```python
from build123d import *

# Parameters (mm, degrees)
SKETCH2_W           = 109
SKETCH2_H           = 114
BOSS_EXTRUDE1_DEPTH = 1.5
SKETCH3_W           = 104
SKETCH3_H           = 109
BOSS_EXTRUDE2_DEPTH = 1
SKETCH4_W           = 25
SKETCH4_H           = 18
CUT_EXTRUDE1_DEPTH  = 2.5


with BuildPart() as part:
    # Sketch2 → Boss-Extrude1 (new body)
    with BuildSketch(Plane(origin=(0, 0, 0), x_dir=(1, 0, 0), z_dir=(0, 1, 0))):
        Rectangle(SKETCH2_W, SKETCH2_H)
    extrude(amount=BOSS_EXTRUDE1_DEPTH)

    # Sketch3 → Boss-Extrude2 (add)
    with BuildSketch(Plane(origin=(0, 1.5, 0), x_dir=(1, 0, 0), z_dir=(0, 1, 0))):
        Rectangle(SKETCH3_W, SKETCH3_H)
    extrude(amount=BOSS_EXTRUDE2_DEPTH)

    # Sketch4 → Cut-Extrude1 (cut)
    with BuildSketch(Plane(origin=(0, 2.5, 0), x_dir=(1, 0, 0), z_dir=(0, 1, 0))):
        with Locations((42, -40.5)):
            Rectangle(SKETCH4_W, SKETCH4_H)
    extrude(amount=-CUT_EXTRUDE1_DEPTH, mode=Mode.SUBTRACT)


solid = part.part
```
Geometry: final body of the model. Coordinates: model frame, mm. A direction names the side the tool comes from. Coordinates: 2 decimals unless noted, no trailing zeros. Loops run counter-clockwise (first coordinate to the right, second up) from the corner with the lowest first, then second, coordinate; pieces in that order, holes last. Notation, with made-up numbers: (53, 34) -> (107, 34) arc R18 ccw to (107, 64) -> close; hole circle Ø11 at (4.25, 9). An arc over 180 degrees is marked (long way). Use a Markdown table: item, result. Add a question column.
(1) Section query A-A, the plane x = 43.5. Return loops of the section in (y, z), plus the area to 3 significant figures.
(2) Section query D-D, the plane x = -2.5. Return loops of the section in (y, z).
(3) Section query B-B, the plane y = 0.7. Return loops of the section in (x, z).
(4) Mould query, pull axis Z, two halves, no side actions, for faces 1 (the flat face through (-53, 1.5, -4)), 2 (the flat face through (42, 1, 49.5)). Classes: pulls with the +Z half, pulls with the -Z half, needs draft (parallel to the pull), parting line crosses it, or undercut.
(5) Pin query (flat end, axial travel): pin 1 Ø0.8 at (x, y) = (37, 2) entering from +Z; pin 2 Ø0.5 at (y, z) = (2, 52.5) entering from +X; pin 3 Ø0.8 at (y, z) = (2, 4) entering from -X. Return the tip coordinate at first contact, or that it passes through.
(6) Section query C-C, the plane z = 37. Return loops of the section in (x, y).
(7) Line query: line 1 along Z through (x, y) = (43.5, 1.7); line 2 along Z through (x, y) = (34, 1.3); line 3 along X through (y, z) = (2.25, 26). Output: solid intervals per line, ascending.
(8) Access query for faces 3 (the flat face through (29.5, 1, 41)), 4 (the flat face through (-1, 0, -1)). Directions: +Z, -Z, +X, -X, +Y, -Y. A direction counts if a zero-diameter tool reaches every point of the face in a straight line with its end or side. Return the directions, or none.
Answer:
| question | item | result |
|---|---|---|
| 1 | outline | (0, -57) -> (1.5, -57) -> (1.5, -54.5) -> (2.5, -54.5) -> (2.5, 31.5) -> (0, 31.5) -> close; (0, 49.5) -> (2.5, 49.5) -> (2.5, 54.5) -> (1.5, 54.5) -> (1.5, 57) -> (0, 57) -> close |
| 1 | area | 235 mm^2 |
| 2 | outline | (0, -57) -> (1.5, -57) -> (1.5, -54.5) -> (2.5, -54.5) -> (2.5, 54.5) -> (1.5, 54.5) -> (1.5, 57) -> (0, 57) -> close |
| 3 | outline | (-54.5, -57) -> (54.5, -57) -> (54.5, 31.5) -> (29.5, 31.5) -> (29.5, 49.5) -> (54.5, 49.5) -> (54.5, 57) -> (-54.5, 57) -> close |
| 4 | face 1 | needs draft |
| 4 | face 2 | undercut |
| 5 | pin 1 | stops at z = 54.5 |
| 5 | pin 2 | stops at x = 52 |
| 5 | pin 3 | stops at x = -52 |
| 6 | outline | (-54.5, 0) -> (29.5, 0) -> (29.5, 2.5) -> (-52, 2.5) -> (-52, 1.5) -> (-54.5, 1.5) -> close |
| 7 | line 1 | z = -54.5 to 31.5, 49.5 to 54.5 |
| 7 | line 2 | z = -57 to 31.5, 49.5 to 57 |
| 7 | line 3 | x = -52 to 52 |
| 8 | face 3 | +X, +Y, -Y |
| 8 | face 4 | +Z, -Z, +X, -X, -Y |
